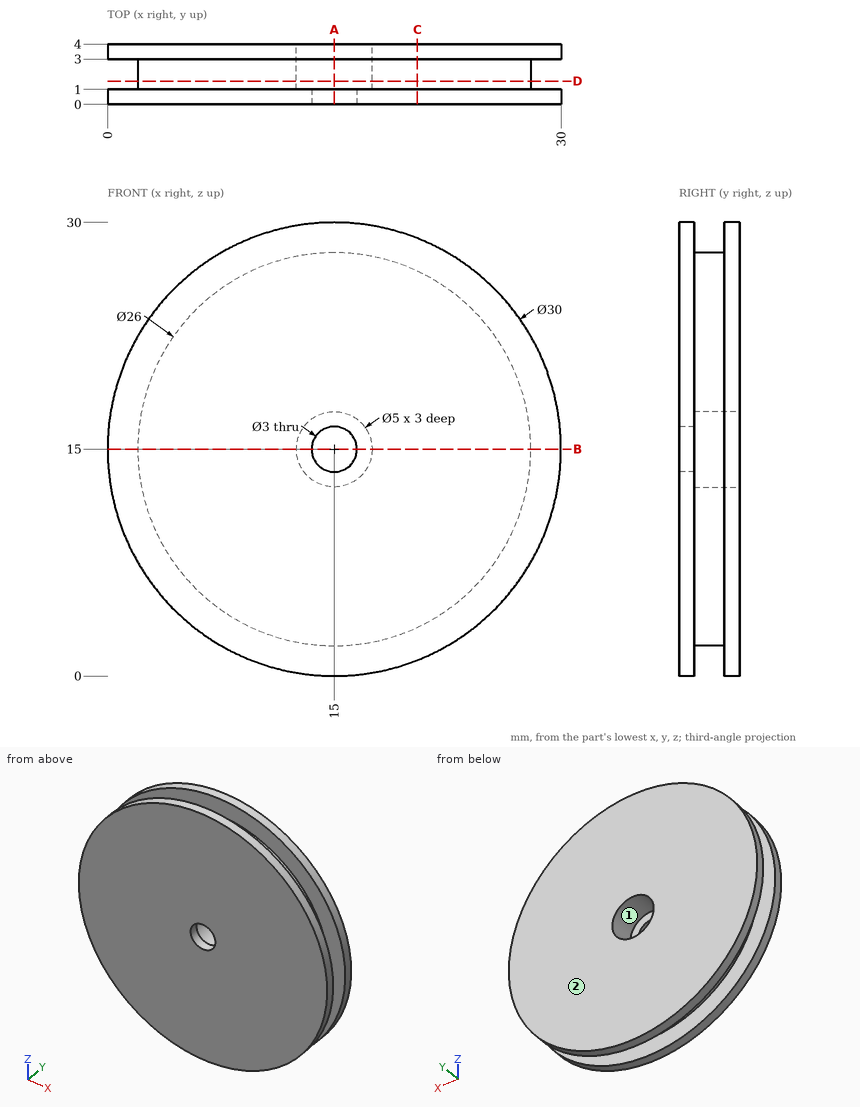
Here's the drawing with two shaded views (mm, measured from the low corner). I have some questions. Give positions to 0.01 mm unless a question says otherwise; leave off trailing zeros. Loops run counter-clockwise (first coordinate to the right, second up) from the corner with the lowest first, then second, coordinate; pieces in that order, holes last. Notation, with made-up numbers: (74.25, 59) - (86.25, 59) arc R24 ccw to (86.25, 86) - close; hole circle Ø4 at (36, -23). An arc over 180 degrees is marked (long way). Answer in a Markdown table with one row per item. Add a question column.
Q1. If we section it at B-B (z = 15): List the corners of the cut face in (x, y) for me, plus the area to 3 significant figures.
Q2. If we section it at C-C (x = 20.5): List the corners of the cut face in (y, z) for me, plus the area to 3 significant figures.
Q3. For pin 1 (4 mm diameter, centred on x = 15, z = 15, fed in from +Y); pin 2 (1.5 mm diameter, centred on y = 1, z = 21, fed in from -X); pin 3 (2 mm diameter, centred on y = 2.5, z = 21.5, fed in from +X), each with a flat end and sliding along its axis, tell me the tip position at first contact or that it passes through.
Q4. If we section it at A-A (x = 15): List the corners of the cut face in (y, z) for me, plus the area to 3 significant figures.
Q5. Please list where these lines run through material, in increasing order: L1, parallel to Z at x = 15, y = 0.75; L2, parallel to Y at x = 20.5, z = 27; L3, parallel to Z at x = 15, y = 1.35. Write a range as from..to.
Q6. If we section it at D-D (y = 1.55): List the corners of the cut face in (x, z) for me, plus the area to 3 significant figures.
Q7. We'd pull the mould along Z, two halves only. Please class the marked faces 1 and 2: +Z half, -Z half, draft (parallel to the pull), parting line (faces both ways), or undercut.
The answers:
| question | item | result |
|---|---|---|
| 1 | outline | (0, 0) - (13.5, 0) - (13.5, 1) - (12.5, 1) - (12.5, 4) - (0, 4) - (0, 3) - (2, 3) - (2, 1) - (0, 1) - close; (16.5, 0) - (30, 0) - (30, 1) - (28, 1) - (28, 3) - (30, 3) - (30, 4) - (17.5, 4) - (17.5, 1) - (16.5, 1) - close |
| 1 | area | 94.0 mm^2 |
| 2 | outline | (0, 1.04) - (1, 1.04) - (1, 3.22) - (3, 3.22) - (3, 1.04) - (4, 1.04) - (4, 28.96) - (3, 28.96) - (3, 26.78) - (1, 26.78) - (1, 28.96) - (0, 28.96) - close |
| 2 | area | 103 mm^2 |
| 3 | pin 1 | stops at y = 1 |
| 3 | pin 2 | stops at x = 0.95 |
| 3 | pin 3 | stops at x = 28.9 |
| 4 | outline | (0, 0) - (1, 0) - (1, 2) - (3, 2) - (3, 0) - (4, 0) - (4, 12.5) - (1, 12.5) - (1, 13.5) - (0, 13.5) - close; (0, 16.5) - (1, 16.5) - (1, 17.5) - (4, 17.5) - (4, 30) - (3, 30) - (3, 28) - (1, 28) - (1, 30) - (0, 30) - close |
| 4 | area | 94.0 mm^2 |
| 5 | L1 | z = 0..13.5, 16.5..30 |
| 5 | L2 | y = 0..1, 3..4 |
| 5 | L3 | z = 2..12.5, 17.5..28 |
| 6 | outline | circle Ø26 at (15, 15); hole circle Ø5 at (15, 15) |
| 6 | area | 511 mm^2 |
| 7 | face 1 | undercut |
| 7 | face 2 | draft |
